Geometry: final body of the model. Coordinates: model frame, mm. Face numbers are marked on the shaded views. A direction names the side the tool comes from. Coordinates: 2 decimals unless noted, no trailing zeros. Order: outer loops, then holes, each group sorted by start corner. A loop starts at its lowest first (then second) coordinate and runs counter-clockwise, first axis right, second up. Notation, with made-up numbers: (24.25, 22.25) - (39.25, 22.25) arc R29 ccw to (39.25, 52.25) - close; hole circle Ø5 at (83.5, 17.25). An arc over 180 degrees is marked (long way). Use one line per item in the form item = value. Start each with the question number.
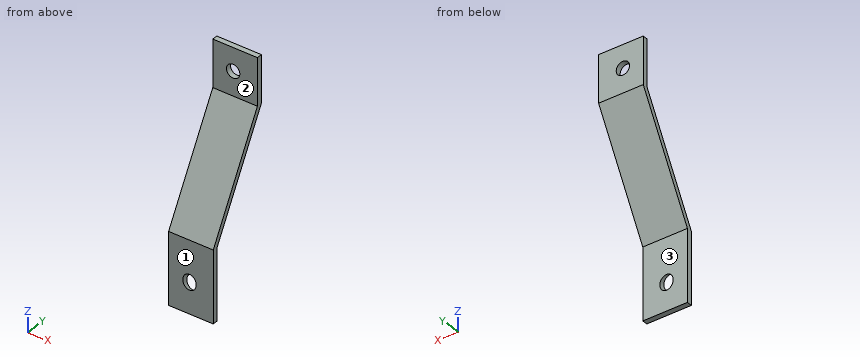
```python
from build123d import *

# Parameters (mm, degrees)
F0_W     = 3.048003
F0_H     = 40.843204
F1_DEPTH = 25.4
F3_D     = 7.62
F5_D     = 7.62


with BuildPart() as f1:
    # F0 (on Right) → F1 (new body)
    with BuildSketch(Plane.YZ):
        Polygon((-15.24, 50.139602), (-49.072802, -10.8204), (-46.024799, -10.8204), (-12.192001, 50.139596), (-12.192001, 76.962002), (-15.24, 76.962002), align=None)
        with Locations((-47.5488, -31.242002)):
            Rectangle(F0_W, F0_H)
    extrude(amount=F1_DEPTH)

    # F3 (through all)
    with Locations(Plane(origin=(0, -32.925578, 18.273696), x_dir=(1, 0, 0), z_dir=(0, -0.874363, 0.485272))):
        with Locations((11.887199, -53.623594)):
            Hole(F3_D / 2)

    # F5 (through all)
    with Locations(Plane.XZ.offset(15.24)):
        with Locations((11.582401, 63.855603)):
            Hole(F5_D / 2)


solid = f1.part
```
(1) Material intervals for L1, parallel to Y at x = 19.5, z = -34.5; L2, parallel to Y at x = 21.5, z = 54; L3, parallel to Z at x = 2, y = -20, sorted ascending. Write a range as from..to.
(2) Cut plane C-C on x = 11. Return the cut outline in (y, z).
(3) Cut plane B-B on z = 62. Return the cut outline in (x, y), plus the area to 3 significant figures.
(4) Cut plane A-A on x = 17. Return the cut outline in (y, z).
(5) Cut plane D-D on y = -31. Return the cut outline in (x, z), plus the area to 3 significant figures.
(6) Set-up query: the marked faces 1, 2 and 3. Return all of +Z, -Z, +X, -X, +Y, -Y with unobstructed straight access to the full face (end or side cutting, diameter ignored); none if empty.
(7) Contact query for flat-ended pins moving along their axis: pin 1 Ø2 at (x, z) = (16.5, -33) entering from +Y; pin 2 Ø1 at (x, y) = (4.5, -18.5) entering from -Z; pin 3 Ø5 at (x, y) = (11.5, -37) entering from +Z; pin 4 Ø4.5 at (x, z) = (11.58, 63.86) entering from -Y. Output: stop coordinate, or through.
Check sheet entries:
q1.L1 = -49.07..-46.02
q1.L2 = -15.24..-12.19
q1.L3 = 36.07..41.56
q2.outline = (-49.07, -51.66) - (-46.02, -51.66) - (-46.02, -40.02) - (-49.07, -38.33) - close; (-49.07, -29.86) - (-46.02, -31.55) - (-46.02, -10.82) - (-12.19, 50.14) - (-12.19, 60.09) - (-15.24, 60.09) - (-15.24, 50.14) - (-49.07, -10.82) - close; (-15.24, 67.62) - (-12.19, 67.62) - (-12.19, 76.96) - (-15.24, 76.96) - close
q3.outline = (0, -15.24) - (8.25, -15.24) - (8.25, -12.19) - (0, -12.19) - close; (14.91, -15.24) - (25.4, -15.24) - (25.4, -12.19) - (14.91, -12.19) - close
q3.area = 57.1 mm^2
q4.outline = (-49.07, -51.66) - (-46.02, -51.66) - (-46.02, -10.82) - (-12.19, 50.14) - (-12.19, 76.96) - (-15.24, 76.96) - (-15.24, 50.14) - (-49.07, -10.82) - close
q5.outline = (0, 16.25) - (25.4, 16.25) - (25.4, 21.74) - (0, 21.74) - close
q5.area = 139 mm^2
q6.face_1 = +Z, -Z, +X, -X, -Y
q6.face_2 = +Z, +X, -X, -Y
q6.face_3 = -Z, +X, -X, +Y
q7.pin_1 = -46.02
q7.pin_2 = 37.87
q7.pin_3 = 15.44
q7.pin_4 = through
